```python
from build123d import *

# Parameters (mm, degrees)
ESQUISSE2_R                  = 52.5
CYLINDRE_DEPTH               = 1000
FENTE_DEPTH                  = 1003.752461977
ESQUISSE4_R                  = 200
SOCLE_DEPTH                  = 50
CORPS_D_PLACER_COPIER1_ANGLE = 180
BOSS_EXTRU_4_START           = 10
ESQUISSE5_R                  = 52.5
BOSS_EXTRU_4_DEPTH           = 10


with BuildPart() as part:
    # Esquisse2 → Cylindre (new body)
    with BuildSketch(Plane(origin=(0, 0, 0), x_dir=(1, 0, 0), z_dir=(0, 1, 0))):
        with Locations(Location((0, 0, 0), (0, 0, 270))):
            Circle(ESQUISSE2_R)
    extrude(amount=CYLINDRE_DEPTH)

    # Esquisse3 → Fente (cut, through all)
    with BuildSketch(Plane(origin=(0, 1000, 0), x_dir=(1, 0, 0), z_dir=(0, 1, 0))):
        with BuildLine():
            Line((0, -52.5), (0, -30))
            ThreePointArc((0, -30), (-2.508787808, -29.894915684), (-5, -29.580398915))
            Line((-5, -29.580398915), (-5, -52.261362401))
            ThreePointArc((-5, -52.261362401), (-2.502845775, -52.440306664), (0, -52.5))
        make_face()
        with BuildLine():
            Line((5, -52.261362401), (5, -29.580398915))
            ThreePointArc((5, -29.580398915), (2.508787808, -29.894915684), (0, -30))
            Line((0, -30), (0, -52.5))
            ThreePointArc((0, -52.5), (2.502845775, -52.440306664), (5, -52.261362401))
        make_face()
    extrude(amount=-FENTE_DEPTH, mode=Mode.SUBTRACT)

    # Esquisse4 → Socle (add)
    with BuildSketch(Plane(origin=(0, 1000, 0), x_dir=(1, 0, 0), z_dir=(0, 1, 0))):
        with Locations(Location((0, 0, 0), (0, 0, 270))):
            Circle(ESQUISSE4_R)
    extrude(amount=SOCLE_DEPTH)


with BuildPart() as part_1:
    # Corps-Déplacer/Copier1: moved
    add(part.part.rotate(Axis((0, 525, 0), (0, 0, 1)), CORPS_D_PLACER_COPIER1_ANGLE))

    # Esquisse5 → Boss.-Extru.4 (add)
    with BuildSketch(Plane(origin=(0, 1050, 0), x_dir=(1, 0, 0), z_dir=(0, 1, 0)).offset(BOSS_EXTRU_4_START)):
        with Locations(Location((0, 0, 0), (0, 0, 180))):
            Circle(ESQUISSE5_R)
    extrude(amount=-BOSS_EXTRU_4_DEPTH)


solid = part_1.part
```
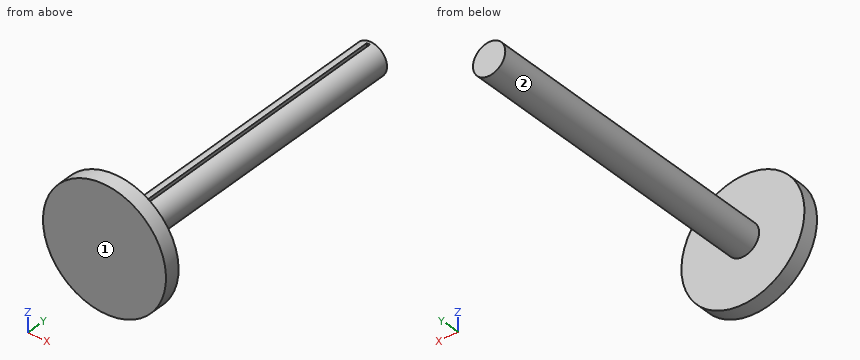
Work out the finished part from the listing and answer in its coordinate system (mm). Face numbers are marked on the shaded views. A direction names the side the tool comes from. Give positions to 0.01 mm unless a question says otherwise; leave off trailing zeros. Loops run counter-clockwise (first coordinate to the right, second up) from the corner with the lowest first, then second, coordinate; pieces in that order, holes last. Notation, with made-up numbers: (8, -20.75) -> (66, -20.75) arc R25 cw to (66, -4.75) -> close; hole circle Ø4 at (-26.75, 66.5). An arc over 180 degrees is marked (long way). One line per question, with ' | ' between items. Start each with the question number.
1) Section A-A, the plane z = 0 is taken. Determine the outline of the cut face in (x, y).
2) Section B-B, the plane y = 682 is taken. Determine the outline of the cut face in (x, z), then the cut area to 3 significant figures.
3) Each of these flat-tipped pins is pushed along its axis until it touches: pin 1 (7 mm diameter, centred on y = 318.5, z = 38.5, fed in from -X); pin 2 (7 mm diameter, centred on y = 388.5, z = 36.5, fed in from +X); pin 3 (1 mm diameter, centred on x = 74, z = -0.5, fed in from +Y). Where does it stop, or does it pass through?
4) Straight lines are drawn through the part: L1, parallel to Y at x = 45.5, z = -172; L2, parallel to X at y = 416.5, z = 15; L3, parallel to Z at x = -8, y = 705. For each, find the intervals that lie inside material, in ascending order.
5) Section D-D, the plane z = 119.5 is taken. Determine the outline of the cut face in (x, y), then the cut area to 3 significant figures.
6) For the marked faces 1 and 2, determine the directions among +Z, -Z, +X, -X, +Y, -Y from which every point of the face is accessible in a straight line to the end or side of a thin tool.
7) Section C-C, the plane x = -71.5 is taken. Determine the outline of the cut face in (y, z).
Resolved:
1) outline: (-200, 0) -> (200, 0) -> (200, 50) -> (52.5, 50) -> (52.5, 1060) -> (-52.5, 1060) -> (-52.5, 50) -> (-200, 50) -> close
2) outline: (-5, 29.58) -> (-5, 52.26) arc R52.5 ccw (long way) to (5, 52.26) -> (5, 29.58) arc R30 ccw to start | area: 8,430 mm2
3) pin 1: x = -39.13 | pin 2: x = 40.83 | pin 3: y = 50
4) L1: 0 to 50 | L2: -50.31 to 50.31 | L3: -51.89 to 51.89
5) outline: (-160.37, 0) -> (160.37, 0) -> (160.37, 50) -> (-160.37, 50) -> close | area: 16,000 mm2
6) face 1: +Z, -Z, +X, -X, -Y | face 2: +Y
7) outline: (0, -186.78) -> (50, -186.78) -> (50, 186.78) -> (0, 186.78) -> close
